Can you work these out from the model? Positions are in its coordinate system, mm. A direction names the side the tool comes from. Round coordinates to 2 decimals unless told otherwise and drop trailing zeros. Loops run counter-clockwise (first coordinate to the right, second up) from the corner with the lowest first, then second, coordinate; pieces in that order, holes last. Notation, with made-up numbers: M 77,7.5 L 126,7.5 A29 cw 126,40.5 Z; hole C -27,36.5 d1. An arc over 180 degrees is marked long. Return JSON: item names as keys, results as strings.
```python
from build123d import *

# Parameters (mm, degrees)
F0_W     = 21
F0_H     = 2
F1_DEPTH = 20.5


with BuildPart() as f1:
    # F0 (on Front) → F1 (new body, symmetric)
    with BuildSketch(Plane.XZ):
        Rectangle(F0_W, F0_H)
        with BuildLine():
            ThreePointArc((-11.667242, 1.609261), (-10.805109, 0.429222), (-10.5, -1))
            Line((-10.5, -1), (-10.5, 1))
            add(Edge.make_bspline(
                [(-10.5, 1), (-10.900594, 1), (-11.368599, 1.342264), (-11.667242, 1.609261)],
                knots=[0, 0, 0, 0, 1.316683, 1.316683, 1.316683, 1.316683], degree=3))
        make_face()
        with BuildLine():
            ThreePointArc((-11.667242, 1.609261), (-17.194891, -2.429222), (-10.5, -1))
            ThreePointArc((-10.5, -1), (-10.805109, 0.429222), (-11.667242, 1.609261))
        make_face()
    extrude(amount=F1_DEPTH, both=True)


solid = f1.part
```
Q1. Suppose I cut it at A-A, the plane x = 6. Please give me the cut outline in (y, z), plus the area to 3 significant figures.
Results:
{"outline": "M -20.5,-1 L 20.5,-1 L 20.5,1 L -20.5,1 Z", "area": "82.0 mm2"}
Q2. On a 3-axis mill with a long thin cutter (end or side, diameter ignored), from which of +Z, -Z, +X, -X, +Y, -Y can I reach the whole of each face in a straight line? I mean faces 1 (the flat face through (-7, -20.5, 0)), 2 (the flat face through (0, 0, -1)), 3 (the flat face through (0, 0, 1)). Say none if no direction works.
Results:
{"face 1": "+Z, -Z, +X, -X, -Y", "face 2": "-Z, +X, +Y, -Y", "face 3": "+Z, +X, +Y, -Y"}
Q3. If I drill on line 1 along Z through (x, y) = (4.75, -7.5); line 2 along X through (y, z) = (14, -1.25); line 3 along X through (y, z) = (-13.5, 0.25), over which ranges is the centre line in solid material (lowest first)?
Results:
{"line 1": "z = -1 to 1", "line 2": "x = -17.49 to -10.51", "line 3": "x = -17.27 to 10.5"}
Q4. Suppose I cut it at B-B, the plane z = -2.75. Please give me the cut outline in (x, y), plus the area to 3 significant figures.
Results:
{"outline": "M -17.03,-20.5 L -10.97,-20.5 L -10.97,20.5 L -17.03,20.5 Z", "area": "249 mm2"}
Q5. I'm going to push flat-ended pins straight in: pin 1 Ø2 at (x, z) = (-3.5, -3.5) entering from +Y; pin 2 Ø6.5 at (x, y) = (3.5, -5.5) entering from -Z; pin 3 Ø12 at (x, y) = (0, -4.5) entering from +Z; pin 4 Ø5 at (x, y) = (-8.5, 3) entering from -Z. Where does each tip first touch, or does it pass through?
Results:
{"pin 1": "passes through", "pin 2": "stops at z = -1", "pin 3": "stops at z = 1", "pin 4": "stops at z = -2.8"}
